Geometry: final body of the model. Coordinates: model frame, mm. A direction names the side the tool comes from. Give positions to 0.01 mm unless a question says otherwise; leave off trailing zeros. Write each loop counter-clockwise with the first axis right and the second up, starting at its lowest first coordinate (ties: lowest second). Pieces come first, ordered by that corner, then holes. Notation, with made-up numbers: (73.5, 81) - (123.5, 81) arc R25 cw to (123.5, 98) - close; hole circle Ø1 at (86.5, 37.25). An arc over 180 degrees is marked (long way). Return JSON: item names as keys, results as strings.
from build123d import *

# Parameters (mm, degrees)
SKETCH3_W            = 241.3
SKETCH3_H            = 228.6
BOSS_EXTRUDE2_DEPTH  = 101.6
SKETCH5_W            = 228.418653982
SKETCH5_H            = 215.9
CUT_EXTRUDE1_DEPTH   = 95.25
FILLET1_R            = 3.175
SKETCH18_R           = 6.35
SKETCH18_R_2         = 12.7
CUT_EXTRUDE5_DEPTH   = 8.89
SKETCH9_R            = 2.54
BOSS_EXTRUDE12_DEPTH = 12.7
SKETCH27_R           = 6.35
CUT_EXTRUDE6_DEPTH   = 8.89


with BuildPart() as part:
    # Sketch3 → Boss-Extrude2 (new body)
    with BuildSketch(Plane(origin=(0, 0, 0), x_dir=(1, 0, 0), z_dir=(0, 1, 0))):
        Rectangle(SKETCH3_W, SKETCH3_H)
    extrude(amount=BOSS_EXTRUDE2_DEPTH)

    # Sketch5 → Cut-Extrude1 (cut)
    with BuildSketch(Plane(origin=(0, 101.6, 0), x_dir=(1, 0, 0), z_dir=(0, 1, 0))):
        Rectangle(SKETCH5_W, SKETCH5_H)
    extrude(amount=-CUT_EXTRUDE1_DEPTH, mode=Mode.SUBTRACT)

    # Fillet1
    fillet1_edges = [part.edges().sort_by_distance(p)[0] for p in [
        (-120.65, 0, 0),
        (0, 0, -114.3),
        (120.65, 0, 0),
        (0, 0, 114.3),
        (-120.65, 50.8, 114.3),
        (-120.65, 50.8, -114.3),
        (120.65, 50.8, -114.3),
        (120.65, 50.8, 114.3),
    ]]
    fillet(fillet1_edges, radius=FILLET1_R)

    # Sketch18 → Cut-Extrude5 (cut)
    with BuildSketch(Plane.XY.offset(-107.95)):
        with Locations((-8.372170426, 25.4)):
            Circle(SKETCH18_R)
        with Locations((-36.121468176, 25.4)):
            Circle(SKETCH18_R_2)
        with Locations((-64.696468176, 25.4)):
            Circle(SKETCH18_R_2)
        with Locations((-93.271468176, 25.4)):
            Circle(SKETCH18_R_2)
        with Locations((-78.983968176, 50.146675913)):
            Circle(SKETCH18_R_2)
        with Locations((-50.408968176, 50.146675913)):
            Circle(SKETCH18_R_2)
    extrude(amount=-CUT_EXTRUDE5_DEPTH, mode=Mode.SUBTRACT)

    # Sketch9 → Boss-Extrude12 (add)
    with BuildSketch(Plane(origin=(0, 6.35, 0), x_dir=(1, 0, 0), z_dir=(0, 1, 0))):
        with Locations(Location((19.467326991, -19.05, 0), (0, 0, 270))):
            Circle(SKETCH9_R)
        with Locations(Location((27.087326991, -19.05, 0), (0, 0, 270))):
            Circle(SKETCH9_R)
        with Locations(Location((-41.492673009, -19.05, 0), (0, 0, 270))):
            Circle(SKETCH9_R)
        with Locations(Location((107.859326991, -19.05, 0), (0, 0, 270))):
            Circle(SKETCH9_R)
        with Locations(Location((107.859326991, 44.45, 0), (0, 0, 270))):
            Circle(SKETCH9_R)
        with Locations(Location((-107.859326991, -101.6, 0), (0, 0, 270))):
            Circle(SKETCH9_R)
        with Locations(Location((-60.234326991, -44.958, 0), (0, 0, 270))):
            Circle(SKETCH9_R)
        with Locations(Location((-107.859326991, -44.958, 0), (0, 0, 270))):
            Circle(SKETCH9_R)
        with Locations(Location((-60.234326991, -101.6, 0), (0, 0, 270))):
            Circle(SKETCH9_R)
        with Locations(Location((-25.512918077, 43.384129, 0), (0, 0, 270))):
            Circle(SKETCH9_R)
        with Locations(Location((-19.924918077, 100.33, 0), (0, 0, 270))):
            Circle(SKETCH9_R)
        with Locations(Location((10.301081923, 43.384129, 0), (0, 0, 270))):
            Circle(SKETCH9_R)
        with Locations(Location((5.475081923, 100.33, 0), (0, 0, 270))):
            Circle(SKETCH9_R)
    extrude(amount=BOSS_EXTRUDE12_DEPTH)

    # Sketch27 → Cut-Extrude6 (cut)
    with BuildSketch(Plane.XY.offset(114.3)):
        with Locations((-39.424308328, 34.84104297)):
            Circle(SKETCH27_R)
        with Locations((106.589326991, 38.1)):
            Circle(SKETCH27_R)
    extrude(amount=-CUT_EXTRUDE6_DEPTH, mode=Mode.SUBTRACT)


solid = part.part
Q1. Section query C-C, the plane x = 88. Return the cut outline in (y, z) (3 decimals).
Answer key:
{"outline": "(0, -111.125) arc R3.175 ccw to (3.175, -114.3) - (101.6, -114.3) - (101.6, -107.95) - (6.35, -107.95) - (6.35, 107.95) - (101.6, 107.95) - (101.6, 114.3) - (3.175, 114.3) arc R3.175 ccw to (0, 111.125) - close"}
Q2. Set-up query: faces 1 (the cylindrical face through (-37.775, 37.992, -111.081)), 2 (the cylindrical face through (-36.011, 40.195, 111.169)), 3 (the flat face through (120.65, 52, 2)), 4 (the flat face through (114.209, 55, 2)), 5 (the flat face through (-120.65, 52, 2)). Return all of +Z, -Z, +X, -X, +Y, -Y with unobstructed straight access to the full face (end or side cutting, diameter ignored); none if empty.
Answer key:
{"face 1": "-Z", "face 2": "+Z", "face 3": "+Z, -Z, +X, +Y, -Y", "face 4": "+Y", "face 5": "+Z, -Z, -X, +Y, -Y"}
Q3. Mould query, pull axis Z, two halves, no side actions, for faces 6 (the flat face through (-2, 6.35, -2)), 7 (the flat face through (-114.209, 55, 2)), 8 (the flat face through (-2, 52, -114.3)), 9 (the cylindrical face through (-94.925, 37.992, -111.081)). Classes: pulls with the +Z half, pulls with the -Z half, needs draft (parallel to the pull), parting line crosses it, or undercut.
Answer key:
{"face 6": "undercut", "face 7": "undercut", "face 8": "pulls with the -Z half", "face 9": "needs draft"}
Q4. Material intervals for probe 1 along X at (y, z) = (25, -111); probe 2 along Z at (x, y) = (-16, 31); probe 3 along X at (y, z) = (51, 45.5), sorted ascending. Write a range as [from, to].
Answer key:
{"probe 1": "x = [-120.65, -105.97], [-80.58, -77.39], [-52, -48.82], [-23.43, -14.71], [-2.03, 120.65]", "probe 2": "z = [-114.3, -107.95], [107.95, 114.3]", "probe 3": "x = [-120.65, -114.21], [114.21, 120.65]"}
Q5. Section query D-D, the plane x = -6.5. Return the cut outline in (y, z) (3 decimals).
Answer key:
{"outline": "(0, -111.125) arc R3.175 ccw to (3.175, -114.3) - (19.332, -114.3) - (19.332, -107.95) - (6.35, -107.95) - (6.35, 107.95) - (101.6, 107.95) - (101.6, 114.3) - (3.175, 114.3) arc R3.175 ccw to (0, 111.125) - close; (31.468, -114.3) - (101.6, -114.3) - (101.6, -107.95) - (31.468, -107.95) - close"}
Q6. Section query A-A, the plane y = 25.4. Return the cut outline in (x, z) (3 decimals).
Answer key:
{"outline": "(-120.65, -111.125) arc R3.175 ccw to (-117.475, -114.3) - (-105.971, -114.3) - (-105.971, -107.95) - (-114.209, -107.95) - (-114.209, 107.95) - (114.209, 107.95) - (114.209, -107.95) - (-2.022, -107.95) - (-2.022, -114.3) - (117.475, -114.3) arc R3.175 ccw to (120.65, -111.125) - (120.65, 111.125) arc R3.175 ccw to (117.475, 114.3) - (-117.475, 114.3) arc R3.175 ccw to (-120.65, 111.125) - close; (-80.571, -114.3) - (-77.396, -114.3) - (-77.396, -107.95) - (-80.571, -107.95) - close; (-51.996, -114.3) - (-48.821, -114.3) - (-48.821, -107.95) - (-51.996, -107.95) - close; (-23.421, -114.3) - (-14.722, -114.3) - (-14.722, -107.95) - (-23.421, -107.95) - close"}
Q7. Section query B-B, the plane z = 69. Return the cut outline in (x, y) (3 decimals).
Answer key:
{"outline": "(-120.65, 3.175) arc R3.175 ccw to (-117.475, 0) - (117.475, 0) arc R3.175 ccw to (120.65, 3.175) - (120.65, 101.6) - (114.209, 101.6) - (114.209, 6.35) - (-114.209, 6.35) - (-114.209, 101.6) - (-120.65, 101.6) - close"}
Q8. Pin query (flat end, axial travel): P1, Ø1.5, axis at x = -26, z = -43.5, coming from the +Y side; P2, Ø5, axis at x = -87, z = -13, coming from the +Y side; P3, Ø23, axis at x = -78.98, y = 50.15, coming from the -Z side. Return the tip coordinate at first contact, or that it passes through.
Answer key:
{"P1": "stops at y = 19.05", "P2": "stops at y = 6.35", "P3": "stops at z = 107.95"}
